Work out the finished part from the listing and answer in its coordinate system (mm). Face numbers are marked on the shaded views. A direction names the side the tool comes from. Coordinates: 2 decimals unless noted, no trailing zeros. Loops run counter-clockwise (first coordinate to the right, second up) from the corner with the lowest first, then second, coordinate; pieces in that order, holes last. Notation, with made-up numbers: M 0.25,83.5 L 31.25,83.5 A19 cw 31.25,115.5 Z; hole C 64.25,-16.5 d1. An arc over 180 degrees is marked long. Write each question's results on one line, items separated by ' | '.
```python
from build123d import *

# Parameters (mm, degrees)
SKETCH1_W           = 1651
SKETCH1_H           = 228.6
BOSS_EXTRUDE1_DEPTH = 228.6
SKETCH2_R           = 63.5
BOSS_EXTRUDE2_DEPTH = 88.9


with BuildPart() as part:
    # Sketch1 → Boss-Extrude1 (new body)
    with BuildSketch(Plane.XY):
        with Locations((825.5, 114.3)):
            Rectangle(SKETCH1_W, SKETCH1_H)
    extrude(amount=BOSS_EXTRUDE1_DEPTH)

    # Sketch2 → Boss-Extrude2 (add)
    with BuildSketch(Plane.XY.offset(228.6)):
        with Locations((190.5, 114.3)):
            Circle(SKETCH2_R)
        with Locations(Location((1460.5, 114.3, 0), (0, 0, 180))):  # turned: the seam where the file's is
            Circle(SKETCH2_R)
    extrude(amount=BOSS_EXTRUDE2_DEPTH)


solid = part.part
```
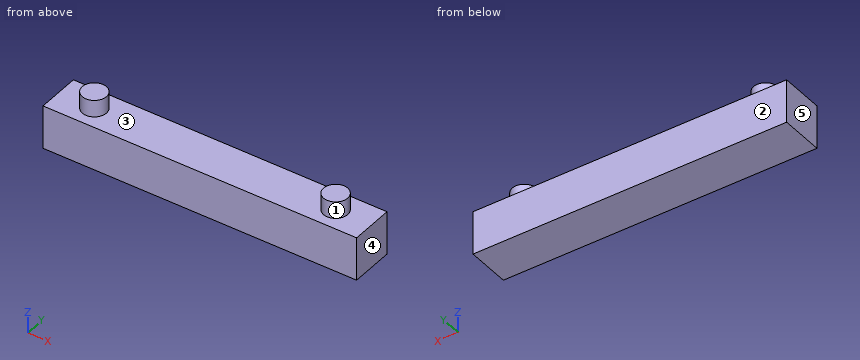
1) Find section C-C, the plane x = 1509.5. Give the vertices of the cut face in (y, z), and give its area (3 significant figures).
Check result:
outline: M 0,0 L 228.6,0 L 228.6,228.6 L 154.69,228.6 L 154.69,317.5 L 73.91,317.5 L 73.91,228.6 L 0,228.6 Z | area: 59,400 mm^2
2) Which of the six approach directions +Z, -Z, +X, -X, +Y, -Y give full straight-line access (tool end or side, diameter ignored) to the marked faces 1 and 2?
Check result:
face 1: +Z | face 2: +Z, -Z, +X, -X, +Y
3) Given pin 1 Ø6 at (y, z) = (145.5, 235) entering from +X; pin 2 Ø6 at (x, y) = (926.5, 98.5) entering from +Z, each flat-ended and moving along its own axis, determine where each tip first touches the part or whether it passes through.
Check result:
pin 1: x = 1517.39 | pin 2: z = 228.6
4) Find section D-D, the plane y = 196. Give the vertices of the cut face in (x, z).
Check result:
outline: M 0,0 L 1651,0 L 1651,228.6 L 0,228.6 Z
5) Straight lines are drawn through the part: probe 1 along Z at (x, y) = (1064, 40.5); probe 2 along X at (y, z) = (148.5, 241.5); probe 3 along X at (y, z) = (153.5, 236). For each, find the intervals that lie inside material, in ascending order. Write a range as [from, to].
Check result:
probe 1: [0, 228.6] | probe 2: [137, 244], [1407, 1514] | probe 3: [140.54, 240.46], [1410.54, 1510.46]
6) For a pull along X with two mould halves and no side action, classify the marked faces 3, 4 and 5 as released by +X, released by -X, zero draft, split by the parting line, or undercut.
Check result:
face 3: undercut | face 4: released by +X | face 5: released by -X
7) Find section B-B, the plane x = 190.5. Give the vertices of the cut face in (y, z).
Check result:
outline: M 0,0 L 228.6,0 L 228.6,228.6 L 177.8,228.6 L 177.8,317.5 L 50.8,317.5 L 50.8,228.6 L 0,228.6 Z
8) Find section A-A, the plane y = 114.3. Give the vertices of the cut face in (x, z), and give its area (3 significant figures).
Check result:
outline: M 0,0 L 1651,0 L 1651,228.6 L 1524,228.6 L 1524,317.5 L 1397,317.5 L 1397,228.6 L 254,228.6 L 254,317.5 L 127,317.5 L 127,228.6 L 0,228.6 Z | area: 400,000 mm^2
